```python
from build123d import *

# Parameters (mm, degrees)
BOSS_EXTRUDE1_DEPTH = 8
SKETCH7_R           = 16.5
BOSS_EXTRUDE2_DEPTH = 8
FILLET1_R           = 0.15


with BuildPart() as part:
    # Sketch1 → Boss-Extrude1 (new body)
    with BuildSketch(Plane.XY):
        with BuildLine():
            Line((-6.5, -15.165750888), (6.5, -15.165750888))
            ThreePointArc((6.5, -15.165750888), (0, 16.5), (-6.5, -15.165750888))
        make_face()
    extrude(amount=-BOSS_EXTRUDE1_DEPTH)

    # Sketch7 → Boss-Extrude2 (add)
    with BuildSketch(Plane(origin=(0, 0, -8), x_dir=(-1, 0, 0), z_dir=(0, 0, -1))):
        Circle(SKETCH7_R)
    extrude(amount=BOSS_EXTRUDE2_DEPTH)

    # Fillet1
    fillet1_edges = [part.edges().sort_by_distance(p)[0] for p in [
        (16.5, 0, -16),
    ]]
    fillet(fillet1_edges, radius=FILLET1_R)


solid = part.part
```
Part model, mm, in its own coordinate system. A direction names the side the tool comes from. Round coordinates to 2 decimals unless told otherwise and drop trailing zeros. Write each loop counter-clockwise with the first axis right and the second up, starting at its lowest first coordinate (ties: lowest second). Pieces come first, ordered by that corner, then holes. Notation, with made-up numbers: (43.5, -35) -> (87.5, -35) arc R28 cw to (87.5, -17) -> close; hole circle Ø3 at (3.5, 4.5). An arc over 180 degrees is marked (long way). Return JSON: item names as keys, results as strings. Group by question number.
Q1. Saw through at C-C on z = -6.25. Write the cut outline in (x, y).
Q2. Saw through at A-A on x = 0. Write the cut outline in (y, z).
Q3. Which spindle directions (+Z, -Z, +X, -X, +Y, -Y) get a long thin tool onto all of the face, cutting with end or side? Do faces 1 (the flat face through (0, -16, -8)), 2 (the flat face through (0, 1, 0)). Say none if no direction does.
Q4. Saw through at B-B on z = -14.5. Write the cut outline in (x, y).
Q5. Pin check, flat tip, straight feed: pin 1 (6.5 mm diameter, centred on x = -1, z = -2.5, fed in from -Y). Stop position of the tip, or through.
Q6. Probe L1, parallel to Y at x = 0, z = -4; L2, parallel to X at y = -12, z = -5.5; L3, parallel to X at y = -1.5, z = -10.25. List the from-to ranges inside material, lowest first. Write a range as [from, to].
Answer:
{
 "1": {"outline": "(-6.5, -15.17) -> (6.5, -15.17) arc R16.5 ccw (long way) to start"},
 "2": {"outline": "(-16.5, -15.85) arc R0.15 ccw to (-16.35, -16) -> (16.35, -16) arc R0.15 ccw to (16.5, -15.85) -> (16.5, 0) -> (-15.17, 0) -> (-15.17, -8) -> (-16.5, -8) -> close"},
 "3": {"face 1": "+Z, +X, -X, -Y", "face 2": "+Z, +X, -X, +Y, -Y"},
 "4": {"outline": "circle Ø33 at (0, 0)"},
 "5": {"pin 1": "y = -15.17"},
 "6": {"L1": "[-15.17, 16.5]", "L2": "[-11.32, 11.32]", "L3": "[-16.43, 16.43]"}
}
